from build123d import *

# Parameters (mm, degrees)
SKETCH025_R  = 11.15
SKETCH025_W  = 10.3
SKETCH025_H  = 2.4
PAD081_DEPTH = 7
PAD083_DEPTH = 16
FILLET005_R  = 3


with BuildPart() as part:
    # Sketch025 → Pad081 (new body)
    with BuildSketch(Plane.XY):
        Circle(SKETCH025_R)
        Rectangle(SKETCH025_W, SKETCH025_H, mode=Mode.SUBTRACT)
    extrude(amount=PAD081_DEPTH)

    # Sketch026 → Pad083 (join)
    with BuildSketch(Plane(origin=(0, 0, 0), x_dir=(-1, 0, 0), z_dir=(0, 0, -1))):
        with BuildLine():
            Line((-5.253749, 7.975), (5.253749, 7.975))
            ThreePointArc((5.253749, -7.975), (9.55, 0), (5.253749, 7.975))
            Line((-5.253749, -7.975), (5.253749, -7.975))
            ThreePointArc((-5.253749, 7.975), (-9.55, 0), (-5.253749, -7.975))
        make_face()
    extrude(amount=PAD083_DEPTH)

    # Fillet005
    fillet005_edges = [part.edges().sort_by_distance(p)[0] for p in [
        (-11.15, 0, 7),
    ]]
    fillet(fillet005_edges, radius=FILLET005_R)


solid = part.part
Geometry check sheet. Reference: the model listing, model coordinates, mm. A direction names the side the tool comes from. Round coordinates to 2 decimals unless told otherwise and drop trailing zeros. Loops run counter-clockwise (first coordinate to the right, second up) from the corner with the lowest first, then second, coordinate; pieces in that order, holes last. Notation, with made-up numbers: (8.25, 60) -> (34.25, 60) arc R16 ccw to (34.25, 88) -> close; hole circle Ø10 at (-28.5, -13). An arc over 180 degrees is marked (long way). Answer as a JSON object with one key per item and string values. Group by question number.
Item 1: Cross-section at C-C, the plane z = -5. Record the cut outline in (x, y) (3 decimals).
Item 2: Depth check by flat-ended pin: pin 1 Ø0.7 at (y, z) = (0.5, 4.5) entering from +X; pin 2 Ø4 at (y, z) = (-6, 3.5) entering from -X; pin 3 Ø6 at (x, z) = (-4.5, 0) entering from +Y. Enter the tip coordinate at first touch or a pass-through.
Item 3: Thickness scan on line 1 along Y through (x, z) = (-1.75, -7) (3 decimals); line 2 along Z through (x, y) = (-4.25, -0.75); line 3 along Y through (x, z) = (1.5, 1.25). Record the ranges inside material, lowest first.
Item 4: Cross-section at B-B, the plane y = 0. Record the cut outline in (x, z).
Item 5: Cross-section at A-A, the plane x = 0. Record the cut outline in (y, z) (3 decimals).
Item 6: Release check for a two-part mould opening along Y. For faces 1 (the face through (0, 7.975, -8)), 2 (the face through (10.635, 3.349, 1.972)), 3 (the face through (-5.15, 0, 3)) record: pulls with the +Y half, pulls with the -Y half, needs draft (parallel to the pull), parting line crosses it, or undercut.
Item 7: Set-up check for faces 4 (the face through (0, -7.975, -8)), 5 (the face through (0, -1.2, 3)), 6 (the face through (-9.55, -0.13, -7.89)): record each of +Z, -Z, +X, -X, +Y, -Y from which the full face is reachable in a straight line by a thin tool's end or side.
Determined:
{
 "1": {"outline": "(-5.254, -7.975) -> (5.254, -7.975) arc R9.55 ccw to (5.254, 7.975) -> (-5.254, 7.975) arc R9.55 ccw to start"},
 "2": {"pin 1": "stops at x = 11.14", "pin 2": "stops at x = -10.41", "pin 3": "stops at y = 11.05"},
 "3": {"line 1": "y = -7.975 to 7.975", "line 2": "z = -16 to 0", "line 3": "y = -11.05 to -1.2, 1.2 to 11.05"},
 "4": {"outline": "(-11.15, 0) -> (-9.55, 0) -> (-9.55, -16) -> (9.55, -16) -> (9.55, 0) -> (11.15, 0) -> (11.15, 4) arc R3 ccw to (8.15, 7) -> (5.15, 7) -> (5.15, 0) -> (-5.15, 0) -> (-5.15, 7) -> (-8.15, 7) arc R3 ccw to (-11.15, 4) -> close"},
 "5": {"outline": "(-11.15, 0) -> (-7.975, 0) -> (-7.975, -16) -> (7.975, -16) -> (7.975, 0) -> (11.15, 0) -> (11.15, 4) arc R3 ccw to (8.15, 7) -> (1.2, 7) -> (1.2, 0) -> (-1.2, 0) -> (-1.2, 7) -> (-8.15, 7) arc R3 ccw to (-11.15, 4) -> close"},
 "6": {"face 1": "pulls with the +Y half", "face 2": "parting line crosses it", "face 3": "undercut"},
 "7": {"face 4": "-Z, +X, -X, -Y", "face 5": "+Z", "face 6": "-Z, -X"}
}
